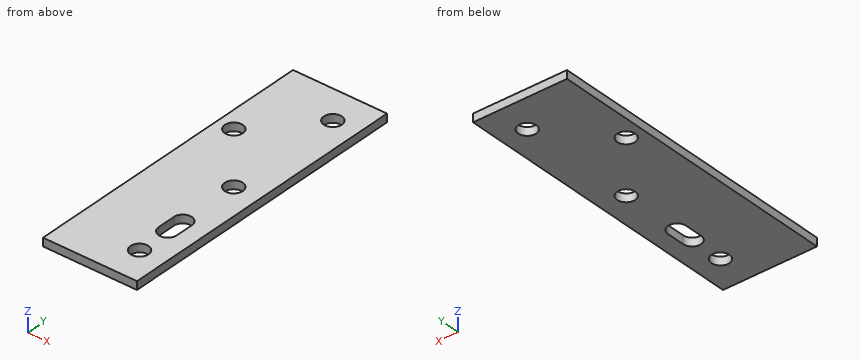
Autodesk Inventor part; units mm, degrees
ref_plane "YZ Plane" through (0, 0, 0) normal (1, 0, 0) x (0, 1, 0)
ref_plane "XZ Plane" through (0, 0, 0) normal (0, 1, 0) x (-1, 0, 0)
ref_plane "XY Plane" through (0, 0, 0) normal (0, 0, 1) x (1, 0, 0)
sketch "Sketch1" plane through (0, 0, 0) normal (0, 0, 1) x (1, 0, 0)
  line L0 (0, 0) -> (35.052, 0)
  line L1 (35.052, 0) -> (35.052, 112.1918)
  line L2 (35.052, 112.1918) -> (0, 112.1918)
  line L3 (0, 112.1918) -> (0, 0)
  dimension "d0" = 35.052
  dimension "d1" = 112.1918
extrude "Plate1" add sketch "Sketch1" along normal blind 3.048
sketch "Sketch2" plane through (0, 0, 3.048) normal (0, 0, 1) x (1, 0, 0)
  circle A0 centre (25.4, 99.4918) radius 3.3655
  circle A1 centre (25.4, 12.7603) radius 3.3655
  circle A2 centre (25.4, 55.0418) radius 3.3655
  circle A3 centre (6.35, 77.978) radius 3.3655
  line L0 (0, 0) -> (0, 112.1918)
  line L1 (28.7655, 32.1818) -> (28.7655, 25.4508)
  line L2 (22.0345, 25.4508) -> (22.0345, 32.1818)
  arc A4 (28.7655, 32.1818) -> (22.0345, 32.1818) centre (25.4, 32.1818) ccw
  line L3 (22.0345, 32.1818) -> (22.0345, 32.1818)
  line L4 (28.7655, 32.1818) -> (28.7655, 32.1818)
  arc A5 (22.0345, 25.4508) -> (28.7655, 25.4508) centre (25.4, 25.4508) ccw
  line L5 (0, 112.1918) -> (35.052, 112.1918)
  line L6 (35.052, 112.1918) -> (35.052, 0)
  point P0 (25.786, 22.1075)
  dimension "hole" = 6.731
  dimension "d42" = 6.731
  dimension "d43" = 6.731
  dimension "d44" = 6.731
  dimension "d49" = 25.4
  dimension "d50" = 6.35
  dimension "d51" = 25.4
  dimension "d54" = 25.4
  dimension "d55" = 44.45
  dimension "d58" = 22.0345
  dimension "d62" = 6.731
  dimension "d63" = 22.86
  dimension "d64" = 12.6905
  dimension "d66" = 25.4
  dimension "d67" = 25.4
  dimension "d68" = 12.7
  dimension "d69" = 21.5138
  dimension "d70" = 3.3655
  dimension "d75" = 9.3472
  dimension "d78" = 6.731
  dimension "d80" = 180
  dimension "d81" = 6.731
extrude "Extrusion1" cut sketch "Sketch2" against normal blind 25.4
equation "\"d42\" = hole"
equation "\"d43\" = hole"
equation "\"d44\" = hole"
equation "\"d70\" = 0.5 * hole"
equation "\"BendRadius\" = Thickness"
equation "\"BendReliefWidth\" = Thickness"
equation "\"BendReliefDepth\" = 0.5 * Thickness"
equation "\"CornerReliefSize\" = 4 * Thickness"
equation "\"MinimumRemnant\" = 2 * Thickness"
equation "\"TransitionRadius\" = BendRadius"
equation "\"JacobiRadiusSize\" = BendRadius"
equation "\"GapSize\" = Thickness"
equation "\"d2\" = BendRadius"
properties part number "Clawplate"
CAD build for the part. Positions are in the model's coordinates, mm. Round coordinates to 2 decimals unless told otherwise and drop trailing zeros. Loops run counter-clockwise (first coordinate to the right, second up) from the corner with the lowest first, then second, coordinate; pieces in that order, holes last. Notation, with made-up numbers: M -32,14 L -17,14 A13 cw -17,36 Z; hole C -17.75,66.5 d5. An arc over 180 degrees is marked long. Use a Markdown table: item, result. Add a question column.
(1) Cut at D-D (z = 0.9). Give the cut face in (x, y), and give its area (3 significant figures).
(2) Drill centre lines: line 1 (Y direction, x = 25.4, z = 2.35); line 2 (Y direction, x = 25, z = 2.55); line 3 (Y direction, x = 7, z = 1.05). Where is each one in solid material? Low to high.
(3) Cut at C-C (y = 34.5). Give the cut face in (x, z).
(4) Cut at B-B (x = 6.35). Give the cut face in (y, z).
(5) Flat gauge pin, fed straight in: pin 1 (6 mm diameter, centred on x = 25.4, y = 55.04, fed in from +Z). Where does the tip first touch, or does it go through?
(6) Cut at A-A (x = 25.4). Give the cut face in (y, z).
Geometry says:
| question | item | result |
|---|---|---|
| 1 | outline | M 0,0 L 35.05,0 L 35.05,112.19 L 0,112.19 Z; hole C 6.35,77.98 d6.73; hole C 25.4,12.76 d6.73; hole M 22.03,25.45 A3.37 ccw 28.77,25.45 L 28.77,32.18 A3.37 ccw 22.03,32.18 Z; hole C 25.4,55.04 d6.73; hole C 25.4,99.49 d6.73 |
| 1 | area | 3,710 mm² |
| 2 | line 1 | y = 0 to 9.39, 16.13 to 22.09, 35.55 to 51.68, 58.41 to 96.13, 102.86 to 112.19 |
| 2 | line 2 | y = 0 to 9.42, 16.1 to 22.11, 35.52 to 51.7, 58.38 to 96.15, 102.83 to 112.19 |
| 2 | line 3 | y = 0 to 74.68, 81.28 to 112.19 |
| 3 | outline | M 0,0 L 22.96,0 L 22.96,3.05 L 0,3.05 Z; M 27.84,0 L 35.05,0 L 35.05,3.05 L 27.84,3.05 Z |
| 4 | outline | M 0,0 L 74.61,0 L 74.61,3.05 L 0,3.05 Z; M 81.34,0 L 112.19,0 L 112.19,3.05 L 81.34,3.05 Z |
| 5 | pin 1 | passes through |
| 6 | outline | M 0,0 L 9.39,0 L 9.39,3.05 L 0,3.05 Z; M 16.13,0 L 22.09,0 L 22.09,3.05 L 16.13,3.05 Z; M 35.55,0 L 51.68,0 L 51.68,3.05 L 35.55,3.05 Z; M 58.41,0 L 96.13,0 L 96.13,3.05 L 58.41,3.05 Z; M 102.86,0 L 112.19,0 L 112.19,3.05 L 102.86,3.05 Z |
